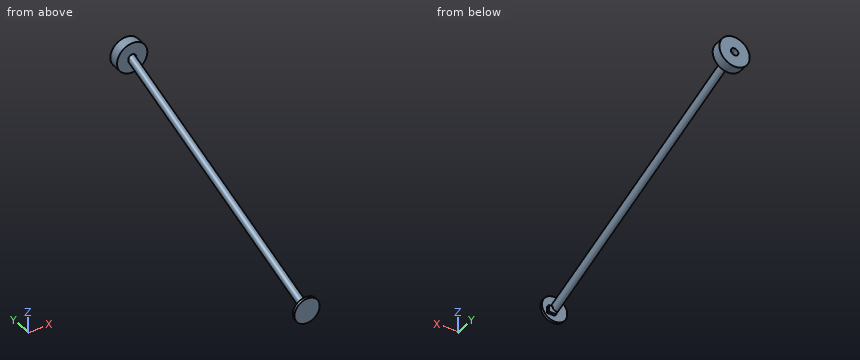
Autodesk Inventor part; units mm, degrees
ref_plane "YZ Plane" through (0, 0, 0) normal (1, 0, 0) x (0, 1, 0)
ref_plane "XZ Plane" through (0, 0, 0) normal (0, 1, 0) x (-1, 0, 0)
ref_plane "XY Plane" through (0, 0, 0) normal (0, 0, 1) x (1, 0, 0)
sketch "Sketch1" plane through (0, 0, 0) normal (0, 1, 0) x (-1, 0, 0)
  circle A0 centre (0, 0) radius 63.5
  dimension "d0" = 127
extrude "Extrusion1" add sketch "Sketch1" along normal blind 12.7
sketch "Sketch2" plane through (0, 12.7, 0) normal (0, 1, 0) x (1, 0, 0)
  circle A0 centre (0, 0) radius 19.05
  circle A1 centre (0, 0) radius 63.5
  line L0 (0, 0) -> (37.718266, 0)
  line L1 (37.718266, 0) -> (37.718266, 33.673151)
  line L2 (37.718266, 33.673151) -> (0, 33.673151)
  line L3 (0, 33.673151) -> (0, 0)
  point P0 (63.5, 0)
  point P1 (0, 19.05)
  point P2 (19.05, 0)
  dimension "d3" = 38.1
extrude "Extrusion2" add sketch "Sketch2" along normal blind 12.7 contours A0 L3 L2 L1 L0
ref_plane "Work Plane1" through (9.525, 12.7, 0) normal (0, -0.9356646, -0.3528907) x (-1, 0, 0)
sketch "Sketch3" plane through (9.525, 12.7, 0) normal (0, -0.9356646, -0.3528907) x (-1, 0, 0)
  circle A0 centre (9.525, -4.481711) radius 19.05
  dimension "d6" = 38.1
extrude "Extrusion3" add sketch "Sketch3" along normal blind 4.826
sketch "Sketch4" plane through (9.525, 12.7, 0) normal (0, 0.9356646, 0.3528907) x (1, 0, 0)
  circle A0 centre (-9.525, -4.481711) radius 19.05
extrude "Extrusion4" add sketch "Sketch4" along normal blind 1422.4
ref_plane "Work Plane2" through (0, 1346.2, 0) normal (0, -1, 0) x (1, 0, 0)
sketch "Sketch5" plane through (0, 1346.2, 0) normal (0, -1, 0) x (1, 0, 0)
  ellipse E0 centre (0, 506.145041) end of major axis (19.05, 506.145041) minor radius 17.82441
  circle A0 centre (0, 506.145041) radius 76.2
  point P0 (0, 0)
  dimension "d12" = 152.4
extrude "Extrusion5" add sketch "Sketch5" along normal blind 25.4 and the other way blind 25.4
properties part number "Legs" material "Aluminum 6061"
Can you work these out from the model? Positions are in its coordinate system, mm. Coordinates: 2 decimals unless noted, no trailing zeros. Write each loop counter-clockwise with the first axis right and the second up, starting at its lowest first coordinate (ties: lowest second). Pieces come first, ordered by that corner, then holes. Notation, with made-up numbers: M 33,20 L 63,20 A29 ccw 63,49 Z; hole C -17.5,40.5 d9. An arc over 180 degrees is marked long. Answer as CSV lines item,"result".
Item 1: Please list where these lines run through material, in increasing order: line 1 along Y through (x, z) = (-16, 534.5); line 2 along Z through (x, y) = (-2, 1204); line 3 along Z through (x, y) = (-16.5, 303.5).
Geometry results:
line 1,"y = 1320.8 to 1371.6"
line 2,"z = 433.85 to 474.34"
line 3,"z = 104.29 to 124.64"
Item 2: I'm going to push flat-ended pins straight in: P1, Ø14, axis at y = 22, z = -27.5, coming from the -X side; P2, Ø6.5, axis at y = 21.5, z = -11, coming from the +X side; P3, Ø5, axis at x = 1.5, y = 1000.5, coming from the +Z side. Where does each tip first touch, or does it pass through?
Geometry results:
P1,"stops at x = 0"
P2,"stops at x = 37.72"
P3,"stops at z = 398.6"
Item 3: Imagine slicing it at A-A on x = -43. List the corners of the cut face in (y, z) for me, plus the area to 3 significant figures.
Geometry results:
outline,"M 0,-46.73 L 12.7,-46.73 L 12.7,46.73 L 0,46.73 Z; M 1320.8,443.24 L 1371.6,443.24 L 1371.6,569.05 L 1320.8,569.05 Z"
area,"7,580 mm2"
